```python
from build123d import *

# Parameters (mm, degrees)
BOSS_EXTRUDE1_DEPTH  = 30
SHELL1_T             = -7
SKETCH2_R            = 15
CUT_EXTRUDE1_DEPTH   = 20
SKETCH3_R            = 2.805999004
CUT_EXTRUDE2_DEPTH   = 20
LPATTERN1_COUNT      = 2
LPATTERN1_PITCH      = 47
LPATTERN1_COUNT_DIR2 = 2
LPATTERN1_PITCH_DIR2 = 47
SKETCH4_R            = 13.106496876
CUT_EXTRUDE3_DEPTH   = 20


with BuildPart() as part:
    # Sketch1 → Boss-Extrude1 (new body)
    with BuildSketch(Plane.XY):
        with BuildLine():
            Line((-98.588677058, 20.737627793), (-48.588677058, 70.737627793))
            Line((-48.588677058, 70.737627793), (30.411322942, 70.737627793))
            ThreePointArc((30.411322942, 70.737627793), (31.118429723, 70.444734574), (31.411322942, 69.737627793))
            Line((31.411322942, 69.737627793), (31.411322942, -49.262372207))
            Line((31.411322942, -49.262372207), (-98.588677058, -49.262372207))
            Line((-98.588677058, -49.262372207), (-98.588677058, 20.737627793))
        make_face()
    extrude(amount=BOSS_EXTRUDE1_DEPTH)

    # Shell1
    shell1_openings = [part.faces().sort_by_distance(p)[0] for p in [
        (-29.379362159, 6.961996775, 30),
    ]]
    offset(amount=SHELL1_T, openings=shell1_openings, kind=Kind.INTERSECTION)

    # Sketch2 → Cut-Extrude1 (cut)
    with BuildSketch(Plane.XY.offset(7)):
        with Locations((-18.588677058, 20.737627793)):
            Circle(SKETCH2_R)
    extrude(amount=-CUT_EXTRUDE1_DEPTH, mode=Mode.SUBTRACT)

    # Sketch3 → Cut-Extrude2 (cut)
    with BuildSketch(Plane.XY.offset(7)):
        with Locations((-42.088677058, 44.237627793)):
            Circle(SKETCH3_R)
    cut_extrude2 = extrude(amount=-CUT_EXTRUDE2_DEPTH, mode=Mode.SUBTRACT)

    # LPattern1: Cut-Extrude2 2 × 2
    with Locations(*[(i * LPATTERN1_PITCH, -j * LPATTERN1_PITCH_DIR2, 0) for i in range(LPATTERN1_COUNT) for j in range(LPATTERN1_COUNT_DIR2) if (i, j) != (0, 0)]):
        add(cut_extrude2, mode=Mode.SUBTRACT)

    # Sketch4 → Cut-Extrude3 (cut)
    with BuildSketch(Plane.XY.offset(7)):
        with Locations((-69.22336781, -8.843391448)):
            Circle(SKETCH4_R)
    extrude(amount=-CUT_EXTRUDE3_DEPTH, mode=Mode.SUBTRACT)


solid = part.part
```
CAD build for the part. Positions are in the model's coordinates, mm. A direction names the side the tool comes from. Round coordinates to 2 decimals unless told otherwise and drop trailing zeros. Order: outer loops, then holes, each group sorted by start corner. A loop starts at its lowest first (then second) coordinate and runs counter-clockwise, first axis right, second up.
Item 1: Tool access for faces 4 (the face through (-33, 12, 0)), 5 (the face through (-33, 11, 7)): list every direction of +Z, -Z, +X, -X, +Y, -Y with a clear straight run to the whole face (end or side of a thin tool).
Item 2: Saw through at D-D on y = -24. Write the cut outline in (x, z), then the cut area to 3 significant figures.
Item 3: Saw through at C-C on x = -23.5. Write the cut outline in (y, z).
Item 4: Saw through at A-A on z = 21. Write the cut outline in (x, y).
Item 5: Mould opens along Y. For faces 1 (the face through (-73.939, 45.388, 14.79)), 2 (the face through (-33, -42.262, 18)), 3 (the face through (31.411, 11, 15)) say: pulls with the +Y half, pulls with the -Y half, needs draft (parallel to the pull), parting line crosses it, or undercut.
Item 6: Probe line 1 along Y through (x, z) = (18.5, 8); line 2 along Y through (x, z) = (-40, 4); line 3 along Y through (x, z) = (-44, 1). List the from-to ranges inside material, lowest first.
Item 7: Saw through at B-B on y = -11. Write the cut outline in (x, z).
Item 8: Pin check, flat tips, straight feed: pin 1 (1.5 mm diameter, centred on x = -63, z = 24.5, fed in from +Y); pin 2 (21 mm diameter, centred on x = -69.22, y = -8.84, fed in from -Z); pin 3 (8 mm diameter, centred on y = 34, z = 11.5, fed in from -X); pin 4 (2 mm diameter, centred on x = -32.5, y = 24, fed in from +Z). Stop position of each tip, or through.
Reported:
1. face 4: -Z, +X, -X, +Y, -Y
1. face 5: +Z
2. outline: (-98.59, 0) - (31.41, 0) - (31.41, 30) - (24.41, 30) - (24.41, 7) - (-91.59, 7) - (-91.59, 30) - (-98.59, 30) - close
2. area: 1,230 mm2
3. outline: (-49.26, 0) - (6.56, 0) - (6.56, 7) - (-42.26, 7) - (-42.26, 30) - (-49.26, 30) - close; (34.91, 0) - (70.74, 0) - (70.74, 30) - (63.74, 30) - (63.74, 7) - (34.91, 7) - close
4. outline: (-98.59, -49.26) - (31.41, -49.26) - (31.41, 69.74) arc R1 ccw to (30.41, 70.74) - (-48.59, 70.74) - (-98.59, 20.74) - close; hole (-91.59, -42.26) - (24.41, -42.26) - (24.41, 63.74) - (-45.69, 63.74) - (-91.59, 17.84) - close
5. face 1: pulls with the +Y half
5. face 2: undercut
5. face 3: needs draft
6. line 1: y = -49.26 to -42.26, 63.74 to 70.74
6. line 2: y = -49.26 to -4.64, -0.89 to 42.36, 46.11 to 70.74
6. line 3: y = -49.26 to -4.82, -0.71 to 42.18, 46.29 to 70.74
7. outline: (-98.59, 0) - (-82.15, 0) - (-82.15, 7) - (-91.59, 7) - (-91.59, 30) - (-98.59, 30) - close; (-56.3, 0) - (31.41, 0) - (31.41, 30) - (24.41, 30) - (24.41, 7) - (-56.3, 7) - close
8. pin 1: stops at y = 57.08
8. pin 2: passes through
8. pin 3: stops at x = -89.33
8. pin 4: stops at z = 7
